```python
from build123d import *

# Parameters (mm, degrees)
SKETCH_2_W                  = 93.1
SKETCH_2_H                  = 10
EXTRUDE_1_DEPTH             = 3.5
SKETCH_4_W                  = 93.1
SKETCH_4_H                  = 6.5
EXTRUDE_2_DEPTH             = 1.1
SKETCH_5_W                  = 93.1
SKETCH_5_H                  = 10
EXTRUDE_3_DEPTH             = 2
CUT_EXTRUDE_1_DEPTH         = 94.867832616
SKETCH_7_W                  = 83.1
SKETCH_7_H                  = 1.1
EXTRUDE_4_DEPTH             = 3.5
CHAMFER_1_SIZE              = 0.4
CUT_EXTRUDE_2_REACH         = 95.868
SKETCH_8_R                  = 150
SKETCH_9_W                  = 93.1
SKETCH_9_H                  = 2
EXTRUDE_5_DEPTH             = 5
EXTRUDE_5_DIRECTION_2_REACH = 95.868
CUT_EXTRUDE_3_REACH         = 95.868
SKETCH_10_W                 = 11.766838493
SKETCH_10_H                 = 1


with BuildPart() as part:
    # 草图2 → 凸台-拉伸1 (new body)
    with BuildSketch(Plane(origin=(0, 0, 0), x_dir=(1, 0, 0), z_dir=(0, 1, 0))):
        with Locations((46.55, 5)):
            Rectangle(SKETCH_2_W, SKETCH_2_H)
    extrude(amount=EXTRUDE_1_DEPTH)

    # 草图4 → 凸台-拉伸2 (add)
    with BuildSketch(Plane(origin=(0, 3.5, 0), x_dir=(1, 0, 0), z_dir=(0, 1, 0))):
        with Locations((46.55, 6.75)):
            Rectangle(SKETCH_4_W, SKETCH_4_H)
    extrude(amount=EXTRUDE_2_DEPTH)

    # 草图5 → 凸台-拉伸3 (add)
    with BuildSketch(Plane(origin=(0, 4.6, 0), x_dir=(1, 0, 0), z_dir=(0, 1, 0))):
        with Locations((46.55, 5)):
            Rectangle(SKETCH_5_W, SKETCH_5_H)
    extrude(amount=EXTRUDE_3_DEPTH)

    # 草图6 → 切除-拉伸1 (cut, through all)
    with BuildSketch(Plane.ZY):
        Polygon((-10, 0), (-6.189488223, 6.6), (-10, 6.6), align=None)
    extrude(amount=-CUT_EXTRUDE_1_DEPTH, mode=Mode.SUBTRACT)

    # 草图7 → 凸台-拉伸4 (add)
    with BuildSketch(Plane.XY.offset(-3.5)):
        with Locations((46.55, 4.05)):
            Rectangle(SKETCH_7_W, SKETCH_7_H)
    extrude(amount=EXTRUDE_4_DEPTH)

    # 倒角1
    chamfer_1_edges = [part.edges().sort_by_distance(p)[0] for p in [
        (90.6, 3.5, 0),
        (2.5, 3.5, 0),
    ]]
    chamfer(chamfer_1_edges, length=CHAMFER_1_SIZE)

    # 草图8 → 切除-拉伸2 (cut, up to next)
    with BuildSketch(Plane.XZ, mode=Mode.PRIVATE) as cut_extrude_2_sk1:
        with Locations((46.55, 147)):
            Circle(SKETCH_8_R)
    cut_extrude_2_tool1 = extrude(cut_extrude_2_sk1.sketch, amount=-CUT_EXTRUDE_2_REACH, mode=Mode.PRIVATE) & part.part
    add(cut_extrude_2_tool1.solids().sort_by_distance((46.55, 0, 147))[0], mode=Mode.SUBTRACT)

    # 草图9 → 凸台-拉伸5 (add)
    with BuildSketch(Plane.XY):
        with Locations((46.55, 5.6)):
            Rectangle(SKETCH_9_W, SKETCH_9_H)
    extrude(amount=EXTRUDE_5_DEPTH)

    # 草图9 → 凸台-拉伸5 direction 2 (add, up to next)
    with BuildSketch(Plane.XY, mode=Mode.PRIVATE) as extrude_5_direction_2_sk1:
        with Locations((46.55, 5.6)):
            Rectangle(SKETCH_9_W, SKETCH_9_H)
    extrude_5_direction_2_tool1 = extrude(extrude_5_direction_2_sk1.sketch, amount=-EXTRUDE_5_DIRECTION_2_REACH, mode=Mode.PRIVATE) - part.part
    add(extrude_5_direction_2_tool1.solids().sort_by_distance((46.55, 5.6, 0))[0])

    # 草图10 → 切除-拉伸3 (cut, up to next)
    with BuildSketch(Plane(origin=(93.1, 0, 0), x_dir=(0, 0, -1), z_dir=(1, 0, 0)), mode=Mode.PRIVATE) as cut_extrude_3_sk1:
        with Locations((0.883419247, 6.1)):
            Rectangle(SKETCH_10_W, SKETCH_10_H)
    cut_extrude_3_tool1 = extrude(cut_extrude_3_sk1.sketch, amount=-CUT_EXTRUDE_3_REACH, mode=Mode.PRIVATE) & part.part
    add(cut_extrude_3_tool1.solids().sort_by_distance((93.1, 6.1, -0.883419))[0], mode=Mode.SUBTRACT)


solid = part.part
```
Design review of the part built by this model. Coordinates are the model's own, in mm. A direction names the side the tool comes from. Coordinates: 2 decimals unless noted, no trailing zeros. Order: outer loops, then holes, each group sorted by start corner. A loop starts at its lowest first (then second) coordinate and runs counter-clockwise, first axis right, second up. Notation, with made-up numbers: (35, -26) - (92, -26) arc R13 ccw to (92, -18) - close; hole circle Ø5 at (-36.75, 8). An arc over 180 degrees is marked (long way). Answer in a Markdown table with one row per item.
(1) Consider section C-C on y = 0.9. State the section outline as (x, z) points.
Checked values:
| item | result |
|---|---|
| outline | (0, -9.48) - (93.1, -9.48) - (93.1, 0) - (76.4, 0) arc R150 cw to (16.7, 0) - (0, 0) - close |
(2) The part is to be moulded in two halves that separate along Y. For faces 1 (the flat face through (91, 3.5, -2)), 2 (the flat face through (85, 2, 0)), 3 (the flat face through (5, 4, -2)), 4 (the flat face through (45.898, 2.761, -8.406)), say which applies: released by +Y, released by -Y, zero draft, split by the parting line, or undercut.
Checked values:
| item | result |
|---|---|
| face 1 | undercut |
| face 2 | zero draft |
| face 3 | undercut |
| face 4 | released by +Y |
(3) Wall thickness on line 1 along Y through (x, z) = (4, 0.25); line 2 along Z through (x, y) = (37, 0.65); line 3 along Z through (x, y) = (71, 3.95): over which ranges is each line inside the solid? List them lowest first. Write a range as from..to.
Checked values:
| item | result |
|---|---|
| line 1 | 4.6..5.6 |
| line 2 | -9.62..-2.7 |
| line 3 | -7.72..-0.99 |
(4) Consider section D-D on z = -9. State the section outline as (x, y) points.
Checked values:
| item | result |
|---|---|
| outline | (0, 0) - (93.1, 0) - (93.1, 1.73) - (0, 1.73) - close |
(5) Clearance check with flat-ended pins moving along their axes: pin 1 (0.9 mm diameter, centred on x = 92, y = 4, fed in from +Z); pin 2 (1.5 mm diameter, centred on x = 44.5, y = 1, fed in from -Z); pin 3 (1.4 mm diameter, centred on x = 82, y = 3, fed in from +Z). State where each tip first meets the part, or that it passes through.
Checked values:
| item | result |
|---|---|
| pin 1 | z = -3.5 |
| pin 2 | z = -9.86 |
| pin 3 | z = 0 |
(6) For faces 5 (the flat face through (88.1, 4, -2)), 6 (the cylindrical face through (46, 2, -3)), 7 (the flat face through (8, 2, 0)), 8 (the flat face through (2, 3.5, -2)), list the 3-axis set-ups (+Z, -Z, +X, -X, +Y, -Y) from which the entire face can be reached by the end or side of a thin tool; tool diameter is ignored.
Checked values:
| item | result |
|---|---|
| face 5 | +Z, +X |
| face 6 | +Z, -Y |
| face 7 | +Z, +X, -X, -Y |
| face 8 | +Z, -X |
(7) Consider section B-B on z = 3.5. State the section outline as (x, y) points, plus the area to 3 significant figures.
Checked values:
| item | result |
|---|---|
| outline | (0, 4.6) - (93.1, 4.6) - (93.1, 5.6) - (0, 5.6) - close |
| area | 93.1 mm^2 |
(8) Consider section A-A on x = 10. State the section outline as (y, z) points, plus the area to 3 significant figures.
Checked values:
| item | result |
|---|---|
| outline | (0, -10) - (5.6, -6.77) - (5.6, 5) - (4.6, 5) - (4.6, 0) - (0, 0) - close |
| area | 51.9 mm^2 |
